Source: CAD feature listing. Evaluate the final solid. Frame: model axes, mm. Face numbers are marked on the shaded views. A direction names the side the tool comes from. Give positions to 0.01 mm unless a question says otherwise; leave off trailing zeros. Write each loop counter-clockwise with the first axis right and the second up, starting at its lowest first coordinate (ties: lowest second). Pieces come first, ordered by that corner, then holes. Notation, with made-up numbers: M -3,46 L 10,46 A23 cw 10,57 Z; hole C 55.25,60 d1. An arc over 180 degrees is marked long. Return JSON: item names as keys, results as strings.
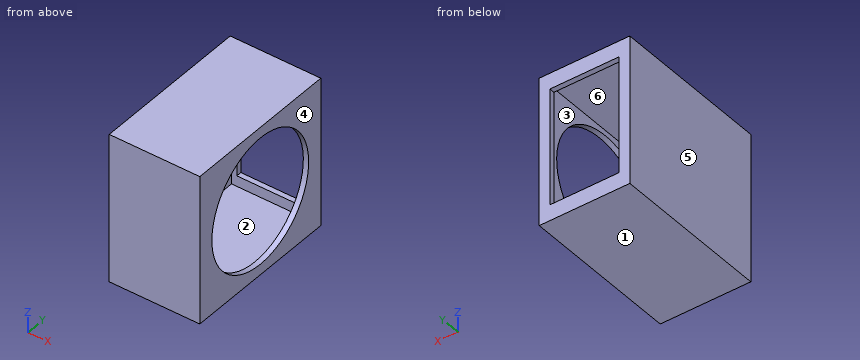
```python
from build123d import *

# Parameters (mm, degrees)
SKETCH1_W           = 8.5
SKETCH1_H           = 15
BOSS_EXTRUDE1_DEPTH = 14
SHELL3_T            = -0.5
SKETCH2_W           = 14
SKETCH2_H           = 15
SKETCH2_R           = 6
BOSS_EXTRUDE2_DEPTH = 0.5
SKETCH3_W           = 6.5
SKETCH3_H           = 11
CUT_EXTRUDE1_DEPTH  = 0.5
SCALE1_SCALE        = 10


with BuildPart() as part:
    # Sketch1 → Boss-Extrude1 (new body)
    with BuildSketch(Plane.XY):
        Rectangle(SKETCH1_W, SKETCH1_H)
    extrude(amount=BOSS_EXTRUDE1_DEPTH)

    # Shell3
    shell3_openings = [part.faces().sort_by_distance(p)[0] for p in [
        (4.25, 0, 7),
    ]]
    offset(amount=SHELL3_T, openings=shell3_openings, kind=Kind.INTERSECTION)

    # Sketch2 → Boss-Extrude2 (add)
    with BuildSketch(Plane(origin=(4.25, 0, 0), x_dir=(0, 0, -1), z_dir=(1, 0, 0))):
        with Locations((-7, 0)):
            Rectangle(SKETCH2_W, SKETCH2_H)
        with Locations((-7, 0)):
            Circle(SKETCH2_R, mode=Mode.SUBTRACT)
    extrude(amount=-BOSS_EXTRUDE2_DEPTH)

    # Sketch3 → Cut-Extrude1 (cut)
    with BuildSketch(Plane(origin=(0, 7.5, 0), x_dir=(1, 0, 0), z_dir=(0, 1, 0))):
        with Locations((0, -7)):
            Rectangle(SKETCH3_W, SKETCH3_H)
    extrude(amount=-CUT_EXTRUDE1_DEPTH, mode=Mode.SUBTRACT)


with BuildPart() as part_1:
    # Scale1: scaled about (-0.690246419, -0.790925988, 7)
    add(part.part.scale(SCALE1_SCALE).moved(Location((6.212217771, 7.118333892, -63))))


solid = part_1.part
```
1) Line query: line 1 (Z direction, x = 15.5, y = -38); line 2 (X direction, y = 10.5, z = 70); line 3 (Y direction, x = 47, z = 7). Output: solid intervals per line, ascending. Write a range as [from, to].
Numbers:
{"line 1": "z = [-63, -58], [72, 77]", "line 2": "x = [-36.29, -31.29], [43.71, 48.71]", "line 3": "y = [-67.88, -52.88], [67.12, 82.12]"}
2) Set-up query: the marked faces 5 and 6. Return all of +Z, -Z, +X, -X, +Y, -Y with unobstructed straight access to the full face (end or side cutting, diameter ignored); none if empty.
Numbers:
{"face 5": "+Z, -Z, -X, +Y, -Y", "face 6": "none"}
3) Cut plane C-C, the plane x = -6.5. Return the cut outline in (y, z), then the cut area to 3 significant figures.
Numbers:
{"outline": "M -67.88,-63 L 82.12,-63 L 82.12,-48 L 77.12,-48 L 77.12,-58 L -62.88,-58 L -62.88,72 L 77.12,72 L 77.12,62 L 82.12,62 L 82.12,77 L -67.88,77 Z", "area": "2,250 mm²"}
4) Draft query along X for the marked faces 1, 2, 3 and 4. Return one class per face: released by +X, released by -X, zero draft, split by the parting line, or undercut.
Numbers:
{"face 1": "zero draft", "face 2": "undercut", "face 3": "undercut", "face 4": "released by +X"}
5) Cut plane D-D, the plane y = 15. Return the cut outline in (x, z), then the cut area to 3 significant figures.
Numbers:
{"outline": "M -36.29,-63 L 48.71,-63 L 48.71,-52.48 L 43.71,-52.48 L 43.71,-58 L -31.29,-58 L -31.29,72 L 43.71,72 L 43.71,66.48 L 48.71,66.48 L 48.71,77 L -36.29,77 Z", "area": "1,560 mm²"}
6) Contact query for flat-ended pins moving along their axis: pin 1 Ø8 at (y, z) = (-8, -3.5) entering from +X; pin 2 Ø12 at (x, z) = (-2.5, -10.5) entering from +Y. Output: stop coordinate, or through.
Numbers:
{"pin 1": "stops at x = -31.29", "pin 2": "stops at y = -62.88"}
7) Cut plane A-A, the plane z = 7. Return the cut outline in (x, y).
Numbers:
{"outline": "M -36.29,-67.88 L 48.71,-67.88 L 48.71,-52.88 L 43.71,-52.88 L 43.71,-62.88 L -31.29,-62.88 L -31.29,77.12 L -26.29,77.12 L -26.29,82.12 L -36.29,82.12 Z; M 38.71,77.12 L 43.71,77.12 L 43.71,67.12 L 48.71,67.12 L 48.71,82.12 L 38.71,82.12 Z"}
8) Cut plane B-B, the plane y = 71. Return the cut outline in (x, z).
Numbers:
{"outline": "M -36.29,-63 L 48.71,-63 L 48.71,77 L -36.29,77 Z; hole M -31.29,-58 L 43.71,-58 L 43.71,72 L -31.29,72 Z"}
